```python
from build123d import *

# Parameters (mm, degrees)
CROQUIS1_W                  = 7.5
CROQUIS1_H                  = 15
CROQUIS1_W_2                = 95
CROQUIS1_H_2                = 3
SALIENTE_EXTRUIR1_DEPTH     = 5
CROQUIS2_W                  = 95
CROQUIS2_H                  = 3
SALIENTE_EXTRUIR2_DEPTH     = 5
CROQUIS5_W                  = 5
CROQUIS5_H                  = 15
CORTAR_EXTRUIR2_DEPTH       = 96.709194961
CROQUIS6_W                  = 5
CROQUIS6_H                  = 23
SALIENTE_EXTRUIR3_DEPTH     = 95
CROQUIS7_W                  = 35
CROQUIS7_H                  = 20
CORTAR_EXTRUIR3_DEPTH       = 52.35659646
CROQUIS9_W                  = 165
CROQUIS9_H                  = 40
SALIENTE_EXTRUIR4_DEPTH     = 50
CROQUIS15_W                 = 95
CROQUIS15_H                 = 15
SALIENTE_EXTRUIR7_DEPTH     = 2
CROQUIS16_R                 = 1.4
CORTAR_EXTRUIR7_DEPTH       = 5
CROQUIS18_W                 = 25
CROQUIS18_H                 = 2
CORTAR_EXTRUIR9_DEPTH       = 5
CORTAR_EXTRUIR10_DEPTH      = 112.719514858
CORTAR_EXTRUIR10_DEPTH_BACK = 43
CROQUIS19_W                 = 140
CROQUIS19_H                 = 25
CROQUIS20_W                 = 10
CROQUIS20_H                 = 35
CROQUIS20_H_2               = 5
CROQUIS20_W_2               = 150
CROQUIS20_W_3               = 5
CORTAR_EXTRUIR11_DEPTH      = 112.719514858
CROQUIS23_W                 = 2
CROQUIS23_H                 = 35
CORTAR_EXTRUIR12_DEPTH      = 163.346080951
CORTAR_EXTRUIR13_DEPTH      = 5
CROQUIS25_W                 = 8
CROQUIS25_H                 = 8
CROQUIS25_W_2               = 5
CROQUIS25_H_2               = 5
SALIENTE_EXTRUIR8_DEPTH     = 5
CROQUIS27_W                 = 5
CROQUIS27_H                 = 3.5
CORTAR_EXTRUIR14_DEPTH      = 5
CROQUIS28_W                 = 8.5
CROQUIS28_H                 = 10
SALIENTE_EXTRUIR9_DEPTH     = 2
CROQUIS29_W                 = 75
CROQUIS29_H                 = 30
CORTAR_EXTRUIR15_DEPTH      = 105.170533262
CROQUIS30_W                 = 8.5
CROQUIS30_H                 = 5
CORTAR_EXTRUIR16_DEPTH      = 7
CROQUIS31_W                 = 18
CROQUIS31_H                 = 25
CORTAR_EXTRUIR17_DEPTH      = 10
CROQUIS32_W                 = 5
CROQUIS32_H                 = 5
CORTAR_EXTRUIR18_DEPTH      = 1
REDONDEO4_R                 = 5


with BuildPart() as part:
    # Croquis1 → Saliente-Extruir1 (new body)
    with BuildSketch(Plane.XY):
        with Locations((43.75, 0)):
            Rectangle(CROQUIS1_W, CROQUIS1_H)
        with Locations((0, 9)):
            Rectangle(CROQUIS1_W_2, CROQUIS1_H_2)
        with Locations((-43.75, 0)):
            Rectangle(CROQUIS1_W, CROQUIS1_H)
    extrude(amount=SALIENTE_EXTRUIR1_DEPTH)

    # Croquis2 → Saliente-Extruir2 (add)
    with BuildSketch(Plane(origin=(0, 0, 0), x_dir=(-1, 0, 0), z_dir=(0, 0, -1))):
        with Locations((0, 9)):
            Rectangle(CROQUIS2_W, CROQUIS2_H)
    extrude(amount=SALIENTE_EXTRUIR2_DEPTH)

    # Croquis5 → Cortar-Extruir2 (cut, through all)
    with BuildSketch(Plane(origin=(47.5, 0, 0), x_dir=(0, 0, -1), z_dir=(1, 0, 0))):
        with Locations((-2.5, 0)):
            Rectangle(CROQUIS5_W, CROQUIS5_H)
    extrude(amount=-CORTAR_EXTRUIR2_DEPTH, mode=Mode.SUBTRACT)

    # Croquis6 → Saliente-Extruir3 (add, through all)
    with BuildSketch(Plane(origin=(47.5, 0, 0), x_dir=(0, 0, -1), z_dir=(1, 0, 0))):
        with Locations((-7.5, -1)):
            Rectangle(CROQUIS6_W, CROQUIS6_H)
    extrude(amount=-SALIENTE_EXTRUIR3_DEPTH)

    # Croquis7 → Cortar-Extruir3 (cut, through all)
    with BuildSketch(Plane.XY.offset(10)):
        with Locations((0, -2.5)):
            Rectangle(CROQUIS7_W, CROQUIS7_H)
    extrude(amount=-CORTAR_EXTRUIR3_DEPTH, mode=Mode.SUBTRACT)

    # Croquis9 → Saliente-Extruir4 (add)
    with BuildSketch(Plane.XY.offset(10)):
        with Locations((-2.5, -32.5)):
            Rectangle(CROQUIS9_W, CROQUIS9_H)
    extrude(amount=-SALIENTE_EXTRUIR4_DEPTH)

    # Croquis15 → Saliente-Extruir7 (add)
    with BuildSketch(Plane(origin=(0, 10.5, 0), x_dir=(1, 0, 0), z_dir=(0, 1, 0))):
        with Locations((0, -2.5)):
            Rectangle(CROQUIS15_W, CROQUIS15_H)
    extrude(amount=SALIENTE_EXTRUIR7_DEPTH)

    # Croquis16 → Cortar-Extruir7 (cut)
    with BuildSketch(Plane(origin=(0, 0, -5), x_dir=(-1, 0, 0), z_dir=(0, 0, -1))):
        with Locations((-37.5, 10)):
            Circle(CROQUIS16_R)
        with Locations(Location((37.5, 10, 0), (0, 0, 180))):
            Circle(CROQUIS16_R)
    extrude(amount=-CORTAR_EXTRUIR7_DEPTH, mode=Mode.SUBTRACT)

    # Croquis18 → Cortar-Extruir9 (cut)
    with BuildSketch(Plane(origin=(0, 12.5, 0), x_dir=(1, 0, 0), z_dir=(0, 1, 0))):
        with Locations((0, -6)):
            Rectangle(CROQUIS18_W, CROQUIS18_H)
    extrude(amount=-CORTAR_EXTRUIR9_DEPTH, mode=Mode.SUBTRACT)

    # Croquis19 → Cortar-Extruir10 (cut, two sides: drawn at the far end of the back side and taken through both)
    with BuildSketch(Plane.XY.offset(10).offset(-CORTAR_EXTRUIR10_DEPTH_BACK)):
        with Locations((0, -30)):
            Rectangle(CROQUIS19_W, CROQUIS19_H)
    extrude(amount=CORTAR_EXTRUIR10_DEPTH + CORTAR_EXTRUIR10_DEPTH_BACK, mode=Mode.SUBTRACT)

    # Croquis20 → Cortar-Extruir11 (cut, through all)
    with BuildSketch(Plane.XY.offset(10)):
        with Locations((-80, -30)):
            Rectangle(CROQUIS20_W, CROQUIS20_H)
        with Locations((-80, -50)):
            Rectangle(CROQUIS20_W, CROQUIS20_H_2)
        with Locations((0, -50)):
            Rectangle(CROQUIS20_W_2, CROQUIS20_H_2)
        with Locations((77.5, -50)):
            Rectangle(CROQUIS20_W_3, CROQUIS20_H_2)
        with Locations((77.5, -30)):
            Rectangle(CROQUIS20_W_3, CROQUIS20_H)
    extrude(amount=-CORTAR_EXTRUIR11_DEPTH, mode=Mode.SUBTRACT)

    # Croquis23 → Cortar-Extruir12 (cut, through all)
    with BuildSketch(Plane(origin=(75, 0, 0), x_dir=(0, 0, -1), z_dir=(1, 0, 0))):
        with Locations((39, -30)):
            Rectangle(CROQUIS23_W, CROQUIS23_H)
    extrude(amount=-CORTAR_EXTRUIR12_DEPTH, mode=Mode.SUBTRACT)

    # Croquis24 → Cortar-Extruir13 (cut)
    with BuildSketch(Plane.ZY.offset(75)):
        Polygon((10, -32.5), (10, -17.5), (-33, -17.5), (-33, -32.5), (-24.5, -32.5), (-24.5, -42.5), (1.5, -42.5), (1.5, -32.5), align=None)
    extrude(amount=-CORTAR_EXTRUIR13_DEPTH, mode=Mode.SUBTRACT)

    # Croquis25 → Saliente-Extruir8 (add, through all)
    with BuildSketch(Plane(origin=(0, -42.5, 0), x_dir=(1, 0, 0), z_dir=(0, 1, 0))):
        with Locations((0, -12.5)):
            Rectangle(CROQUIS25_W, CROQUIS25_H)
        with Locations((0, -12.5)):
            Rectangle(CROQUIS25_W_2, CROQUIS25_H_2, mode=Mode.SUBTRACT)
    extrude(amount=-SALIENTE_EXTRUIR8_DEPTH)

    # Croquis27 → Cortar-Extruir14 (cut)
    with BuildSketch(Plane(origin=(0, -12.5, 0), x_dir=(1, 0, 0), z_dir=(0, 1, 0))):
        with Locations((0, -6.75)):
            Rectangle(CROQUIS27_W, CROQUIS27_H)
    extrude(amount=-CORTAR_EXTRUIR14_DEPTH, mode=Mode.SUBTRACT)

    # Croquis28 → Saliente-Extruir9 (add)
    with BuildSketch(Plane(origin=(-70, 0, 0), x_dir=(0, 0, -1), z_dir=(1, 0, 0))):
        with Locations((-5.75, -37.5)):
            Rectangle(CROQUIS28_W, CROQUIS28_H)
        with Locations((28.75, -37.5)):
            Rectangle(CROQUIS28_W, CROQUIS28_H)
    extrude(amount=SALIENTE_EXTRUIR9_DEPTH)

    # Croquis29 → Cortar-Extruir15 (cut, through all)
    with BuildSketch(Plane.XY.offset(16.5)):
        with Locations((0, -32.5)):
            Rectangle(CROQUIS29_W, CROQUIS29_H)
    extrude(amount=-CORTAR_EXTRUIR15_DEPTH, mode=Mode.SUBTRACT)

    # Croquis30 → Cortar-Extruir16 (cut)
    with BuildSketch(Plane.ZY.offset(75)):
        with Locations((5.75, -35)):
            Rectangle(CROQUIS30_W, CROQUIS30_H)
    extrude(amount=-CORTAR_EXTRUIR16_DEPTH, mode=Mode.SUBTRACT)

    # Croquis31 → Cortar-Extruir17 (cut)
    with BuildSketch(Plane.XY.offset(10)):
        with Locations((-38.5, 0)):
            Rectangle(CROQUIS31_W, CROQUIS31_H)
    extrude(amount=-CORTAR_EXTRUIR17_DEPTH, mode=Mode.SUBTRACT)

    # Croquis32 → Cortar-Extruir18 (cut)
    with BuildSketch(Plane.ZY.offset(47.5)):
        with Locations((-2.5, 10)):
            Rectangle(CROQUIS32_W, CROQUIS32_H)
    extrude(amount=-CORTAR_EXTRUIR18_DEPTH, mode=Mode.SUBTRACT)

    # Redondeo4
    redondeo4_edges = [part.edges().sort_by_distance(p)[0] for p in [
        (-29.5, 0, 10),
    ]]
    fillet(redondeo4_edges, radius=REDONDEO4_R)


solid = part.part
```
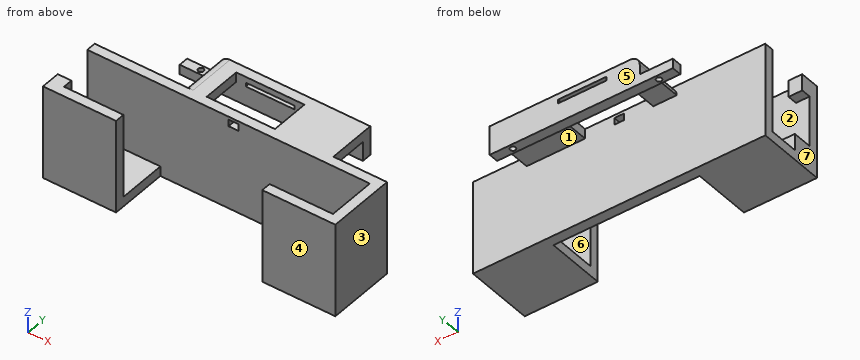
Verification items for the finished model (mm, model axes). Face numbers are marked on the shaded views. A direction names the side the tool comes from. Coordinates: 2 decimals unless noted, no trailing zeros. Write each loop counter-clockwise with the first axis right and the second up, starting at its lowest first coordinate (ties: lowest second). Pieces come first, ordered by that corner, then holes. Notation, with made-up numbers: (16, 63.25) - (28, 63.25) arc R12 ccw to (28, 83.25) - close; hole circle Ø11 at (68, 16). An arc over 180 degrees is marked (long way). One line per question, with ' | ' between items. Start each with the question number.
1. Section check C-C (y = 10). Enter the section's corners in (x, z).
2. Gauge pin test, flat ends, axial feed: P1, Ø6, axis at x = 56, y = -31.5, coming from the +Z side; P2, Ø8, axis at x = 17.5, z = -10, coming from the +Y side; P3, Ø14.5, axis at x = 2, z = -23.5, coming from the -Y side; P4, Ø2.5, axis at x = -37.5, y = 10, coming from the -Z side. Record the tip position at first contact, or that the pin passes through.
3. Section check D-D (y = -28). Enter the section's corners in (x, z), plus the area to 3 significant figures.
4. Access from +Z, -Z, +X, -X, +Y, -Y to the whole of each face (thin tool, end or side, straight path). Record for the marked faces 1, 2 and 3.
5. Section check B-B (x = 9). Enter the section's corners in (y, z).
6. Draft check along Y on the marked faces 4, 5, 6 and 7. Enter one of: released by +Y, released by -Y, zero draft, split by the parting line, or undercut.
7. Section check A-A (z = -30). Enter the section's corners in (x, y), plus the area to 3 significant figures.
8. Material ranges on line 1 along Y through (x, z) = (44, -10); line 2 along X through (y, z) = (-44, 6); line 3 along Z through (x, y) = (46, -27), recorded low to high.
Computed values:
1) outline: (-46.5, -5) - (-38.9, -5) - (-38.9, 0) - (-46.5, 0) - close; (-36.1, -5) - (36.1, -5) - (36.1, 0) - (38.9, 0) - (38.9, -5) - (47.5, -5) - (47.5, 10) - (-24.5, 10) arc R5 ccw to (-29.5, 5) - (-29.5, 0) - (-36.1, 0) - close; hole (-12.5, 5) - (12.5, 5) - (12.5, 7) - (-12.5, 7) - close
2) P1: z = -33 | P2: y = -12.5 | P3: y = -17.5 | P4: through
3) outline: (-75, -38) - (-37.5, -38) - (-37.5, -33) - (-75, -33) - close; (37.5, -38) - (75, -38) - (75, 10) - (70, 10) - (70, -33) - (37.5, -33) - close | area: 590 mm²
4) face 1: -Z, +X, -X | face 2: none | face 3: +Z, -Z, +X, +Y, -Y
5) outline: (-17.5, -38) - (-12.5, -38) - (-12.5, 10) - (-17.5, 10) - close; (7.5, -5) - (12.5, -5) - (12.5, 5) - (7.5, 5) - close; (7.5, 7) - (12.5, 7) - (12.5, 10) - (7.5, 10) - close
6) face 4: released by -Y | face 5: released by +Y | face 6: undercut | face 7: zero draft
7) outline: (-75, -47.5) - (-37.5, -47.5) - (-37.5, -42.5) - (-68, -42.5) - (-68, -32.5) - (-75, -32.5) - close; (-75, -17.5) - (70, -17.5) - (70, -42.5) - (37.5, -42.5) - (37.5, -47.5) - (75, -47.5) - (75, -12.5) - (-75, -12.5) - close | area: 1,320 mm²
8) line 1: -47.5 to -42.5, -17.5 to -12.5 | line 2: -75 to -37.5, 37.5 to 75 | line 3: -38 to -33
